Verification items for the finished model (mm, model axes). Give positions to 0.01 mm unless a question says otherwise; leave off trailing zeros. Loops run counter-clockwise (first coordinate to the right, second up) from the corner with the lowest first, then second, coordinate; pieces in that order, holes last. Notation, with made-up numbers: (5, 56.25) - (42, 56.25) arc R23 ccw to (42, 87.25) - close; hole circle Ø11 at (1, 64.5). An arc over 180 degrees is marked (long way). One line per item, written item: value. Start each with the question number.
1. Sectioned sample at D-D (y = 1.05). Record the cut outline in (x, z).
2. Scan lines: L1, parallel to X at y = 1.75, z = 10; L2, parallel to X at y = 0.9, z = -4; L3, parallel to Z at x = -22, y = 0.3. Record each from-to range of solid material in increasing order. Write a range as [from, to].
3. Gauge pin test, flat end, axial feed: pin 1 (5 mm diameter, centred on x = 20, z = 10, fed in from -Y). Record the tip position at first contact, or that the pin passes through.
4. Sectioned sample at A-A (z = 0.75). Record the cut outline in (x, y), plus the area to 3 significant figures.
5. Sectioned sample at C-C (x = -20). Record the cut outline in (y, z).
6. Sectioned sample at B-B (z = -10). Record the cut outline in (x, y), plus the area to 3 significant figures.
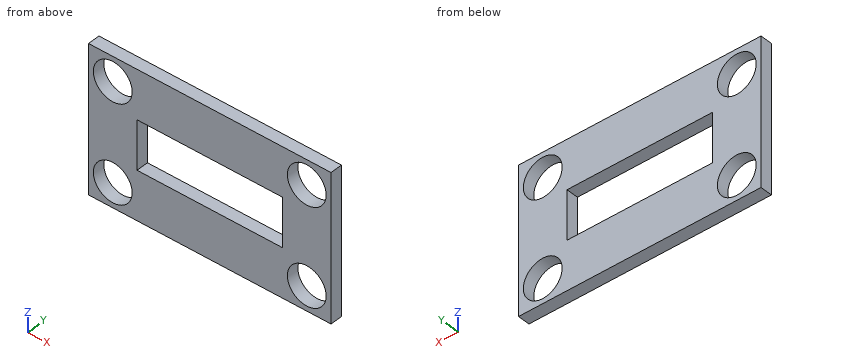
from build123d import *

# Parameters (mm, degrees)
SKETCH2_W           = 50
SKETCH2_H           = 30
SKETCH2_R           = 4
BOSS_EXTRUDE1_DEPTH = 2.5
SKETCH3_W           = 30
SKETCH3_H           = 10
CUT_EXTRUDE1_DEPTH  = 5


with BuildPart() as part:
    # Sketch2 → Boss-Extrude1 (new body)
    with BuildSketch(Plane(origin=(0, 0, 0), x_dir=(1, 0, 0), z_dir=(0, 1, 0))):
        Rectangle(SKETCH2_W, SKETCH2_H)
        with Locations(Location((-20, -10, 0), (0, 0, 270))):
            Circle(SKETCH2_R, mode=Mode.SUBTRACT)
        with Locations(Location((20, -10, 0), (0, 0, 270))):
            Circle(SKETCH2_R, mode=Mode.SUBTRACT)
        with Locations(Location((20, 10, 0), (0, 0, 270))):
            Circle(SKETCH2_R, mode=Mode.SUBTRACT)
        with Locations(Location((-20, 10, 0), (0, 0, 270))):
            Circle(SKETCH2_R, mode=Mode.SUBTRACT)
    extrude(amount=BOSS_EXTRUDE1_DEPTH)

    # Sketch3 → Cut-Extrude1 (cut)
    with BuildSketch(Plane(origin=(0, 2.5, 0), x_dir=(1, 0, 0), z_dir=(0, 1, 0))):
        Rectangle(SKETCH3_W, SKETCH3_H)
    extrude(amount=-CUT_EXTRUDE1_DEPTH, mode=Mode.SUBTRACT)


solid = part.part
Results are:
1. outline: (-25, -15) - (25, -15) - (25, 15) - (-25, 15) - close; hole circle Ø8 at (-20, -10); hole circle Ø8 at (-20, 10); hole (-15, -5) - (15, -5) - (15, 5) - (-15, 5) - close; hole circle Ø8 at (20, -10); hole circle Ø8 at (20, 10)
2. L1: x = [-25, -24], [-16, 16], [24, 25]
2. L2: x = [-25, -15], [15, 25]
2. L3: z = [-15, -13.46], [-6.54, 6.54], [13.46, 15]
3. pin 1: passes through
4. outline: (-25, 0) - (-15, 0) - (-15, 2.5) - (-25, 2.5) - close; (15, 0) - (25, 0) - (25, 2.5) - (15, 2.5) - close
4. area: 50.0 mm^2
5. outline: (0, -15) - (2.5, -15) - (2.5, -14) - (0, -14) - close; (0, -6) - (2.5, -6) - (2.5, 6) - (0, 6) - close; (0, 14) - (2.5, 14) - (2.5, 15) - (0, 15) - close
6. outline: (-25, 0) - (-24, 0) - (-24, 2.5) - (-25, 2.5) - close; (-16, 0) - (16, 0) - (16, 2.5) - (-16, 2.5) - close; (24, 0) - (25, 0) - (25, 2.5) - (24, 2.5) - close
6. area: 85.0 mm^2
